Source: three-view drawing plus pictorial views. Frame: mm from the lowest corner of the part. Coordinates: 2 decimals unless noted, no trailing zeros. Write each loop counter-clockwise with the first axis right and the second up, starting at its lowest first coordinate (ties: lowest second). Pieces come first, ordered by that corner, then holes. Notation, with made-up numbers: (-13, -17) -> (12, -17) arc R22 ccw to (12, 2) -> close; hole circle Ø1 at (58, 35). An arc over 180 degrees is marked (long way). One line per item, written item: value.
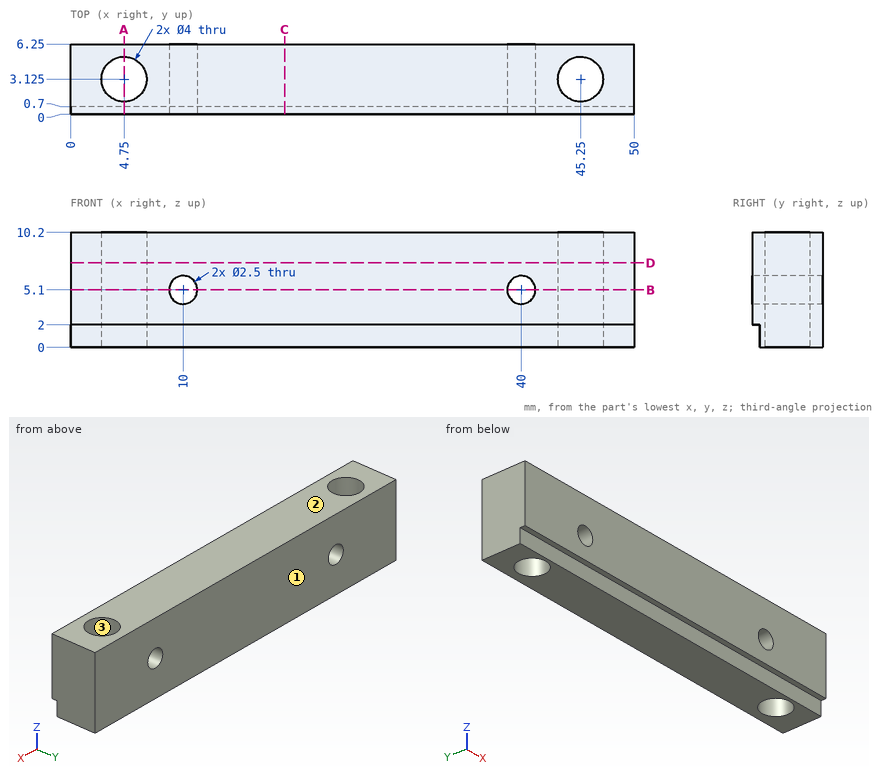
(1) Section B-B (z = 5.1). Return the cut outline in (x, y) (3 decimals).
Responses:
outline: (0, 0) -> (8.75, 0) -> (8.75, 6.25) -> (0, 6.25) -> close; (11.25, 0) -> (38.75, 0) -> (38.75, 6.25) -> (11.25, 6.25) -> close; (41.25, 0) -> (50, 0) -> (50, 6.25) -> (41.25, 6.25) -> close; hole circle Ø4 at (4.75, 3.125); hole circle Ø4 at (45.25, 3.125)
(2) Section A-A (x = 4.75). Return the cut outline in (y, z) (3 decimals), then the cut area to 4 significant figures.
Responses:
outline: (0, 2) -> (0.7, 2) -> (0.7, 0) -> (1.125, 0) -> (1.125, 10.2) -> (0, 10.2) -> close; (5.125, 0) -> (6.25, 0) -> (6.25, 10.2) -> (5.125, 10.2) -> close
area: 21.55 mm2
(3) Line query: line 1 (X direction, y = 4.25, z = 6.5); line 2 (X direction, y = 4, z = 6.5); line 3 (X direction, y = 4.5, z = 4.75). Output: solid intervals per line, ascending. Write a range as [from, to].
Responses:
line 1: x = [0, 3.1], [6.4, 43.6], [46.9, 50]
line 2: x = [0, 2.95], [6.55, 43.45], [47.05, 50]
line 3: x = [0, 3.3], [6.2, 8.8], [11.2, 38.8], [41.2, 43.8], [46.7, 50]
(4) Section C-C (x = 19). Return the cut outline in (y, z), then the cut area to 4 significant figures.
Responses:
outline: (0, 2) -> (0.7, 2) -> (0.7, 0) -> (6.25, 0) -> (6.25, 10.2) -> (0, 10.2) -> close
area: 62.35 mm2
(5) Section D-D (z = 7.5). Return the cut outline in (x, y) (3 decimals), then the cut area to 3 significant figures.
Responses:
outline: (0, 0) -> (50, 0) -> (50, 6.25) -> (0, 6.25) -> close; hole circle Ø4 at (4.75, 3.125); hole circle Ø4 at (45.25, 3.125)
area: 287 mm2
(6) First-contact query: pin 1 (2 mm diameter, centred on y = 1.5, z = 2.5, fed in from -X). Flat tip, straight axial feed; report the tip coordinate or a pass-through.
Responses:
pin 1: stops at x = 0
(7) Pull-direction query (Y, two-part tool) for the marked faces 1, 2 and 3; classes: released by +Y, released by -Y, zero draft, split by the parting line, or undercut.
Responses:
face 1: released by +Y
face 2: zero draft
face 3: undercut
